Part model, mm, in its own coordinate system. Face numbers are marked on the shaded views. A direction names the side the tool comes from. Give positions to 0.01 mm unless a question says otherwise; leave off trailing zeros. Write each loop counter-clockwise with the first axis right and the second up, starting at its lowest first coordinate (ties: lowest second). Pieces come first, ordered by that corner, then holes. Notation, with made-up numbers: (3, 3) - (13, 3) arc R9 cw to (13, 12) - close; hole circle Ø6 at (28.25, 61.25). An arc over 180 degrees is marked (long way). Answer as a JSON object with one key per item and string values. Group by question number.
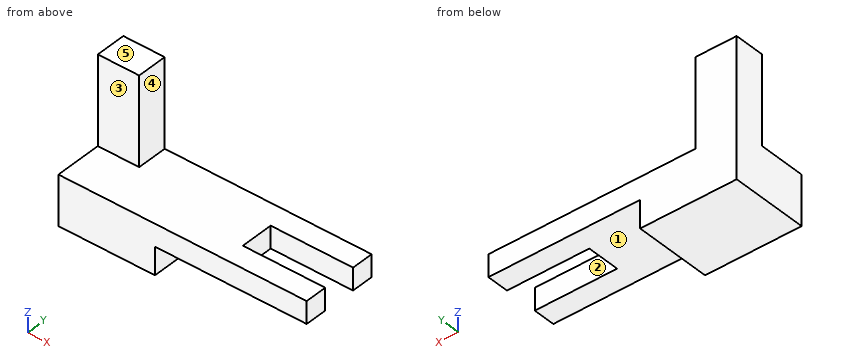
```python
from build123d import *

# Parameters (mm, degrees)
F1_DEPTH = 28
F2_W     = 17
F2_H     = 32
F3_DEPTH = 25
F4_W     = 29.857718
F4_H     = 12
F5_DEPTH = 25


with BuildPart() as f1:
    # F0 (on Front) → F1 (new body)
    with BuildSketch(Plane.XZ):
        Polygon((0, 50), (0, 0), (35, 0), (35, 10), (90, 10), (90, 18), (15, 18), (15, 50), align=None)
    extrude(amount=F1_DEPTH)

    # F2 (on face) → F3 (cut)
    with BuildSketch(Plane.YZ.offset(15)):
        with Locations((-19.5, 34)):
            Rectangle(F2_W, F2_H)
    extrude(amount=-F3_DEPTH, mode=Mode.SUBTRACT)

    # F4 (on face) → F5 (cut)
    with BuildSketch(Plane.XY.offset(18)):
        with Locations((75.071141, -14)):
            Rectangle(F4_W, F4_H)
    extrude(amount=-F5_DEPTH, mode=Mode.SUBTRACT)


solid = f1.part
```
1) Band-saw the part on B-B (y = -26.5). List the corners of the cut face in (x, z), plus the area to 3 significant figures.
2) Which spindle directions (+Z, -Z, +X, -X, +Y, -Y) get a long thin tool onto all of the face, cutting with end or side? Do the marked faces 1, 2, 3, 4 and 5. Say none if no direction does.
3) Band-saw the part on D-D (x = 56). List the corners of the cut face in (y, z).
4) Drop flat-ended pins along their axis: P1, Ø2.5, axis at y = -14.5, z = 13, coming from the +X side; P2, Ø1.5, axis at y = -12, z = 27.5, coming from the -X side; P3, Ø9, axis at y = -4.5, z = 28, coming from the +X side; P4, Ø12, axis at x = 10, z = 28.5, coming from the -Y side. Give the stop position or say it passes through.
5) Band-saw the part on C-C (z = 9). List the corners of the cut face in (x, y).
6) Band-saw the part on A-A (x = 80.5). List the corners of the cut face in (y, z), plus the area to 3 significant figures.
7) Probe line 1 (Z direction, x = 58.5, y = -5.25); line 2 (Z direction, x = 23, y = -11.25); line 3 (X direction, y = -14.75, z = 8). List the from-to ranges inside material, lowest first.
Verdict:
{
 "1": {"outline": "(0, 0) - (35, 0) - (35, 10) - (90, 10) - (90, 18) - (0, 18) - close", "area": "1,070 mm2"},
 "2": {"face 1": "-Z, +X, +Y, -Y", "face 2": "+Z, -Z, +X", "face 3": "+Z, +X, -X, -Y", "face 4": "+Z, +X, +Y, -Y", "face 5": "+Z, +X, -X, +Y, -Y"},
 "3": {"outline": "(-28, 10) - (0, 10) - (0, 18) - (-28, 18) - close"},
 "4": {"P1": "x = 60.14", "P2": "through", "P3": "x = 15", "P4": "y = -11"},
 "5": {"outline": "(0, -28) - (35, -28) - (35, 0) - (0, 0) - close"},
 "6": {"outline": "(-28, 10) - (-20, 10) - (-20, 18) - (-28, 18) - close; (-8, 10) - (0, 10) - (0, 18) - (-8, 18) - close", "area": "128 mm2"},
 "7": {"line 1": "10 to 18", "line 2": "0 to 18", "line 3": "0 to 35"}
}
